from build123d import *

# Parameters (mm, degrees)
F0_W     = 76.2
F0_H     = 50.8
F0_R     = 12.7
F1_DEPTH = 12.7
F2_W     = 6.35
F2_H     = 50.8
F3_DEPTH = 2.54
F5_DEPTH = 58
F6_R     = 3.175
F7_DEPTH = 12.7


# Not quite as in the source:
# - a feature names something its author has since deleted; it is built from what else it names


with BuildPart() as f1:
    # F0 (on Top) → F1 (new body)
    with BuildSketch(Plane.XY):
        with Locations((-0.2381126344, 0.8489250481)):
            Rectangle(F0_W, F0_H)
        Circle(F0_R, mode=Mode.SUBTRACT)
    extrude(amount=F1_DEPTH)

    # F2 (on face) → F3 (cut)
    with BuildSketch(Plane.XY.offset(12.7)):
        with BuildLine():
            Line((6.35, 26.2489250481), (-6.35, 26.2489250481))
            Line((-6.35, 26.2489250481), (-6.35, 10.9985226281))
            ThreePointArc((-6.35, 10.9985226281), (0, 12.7), (6.35, 10.9985226281))
            Line((6.35, 10.9985226281), (6.35, 26.2489250481))
        make_face()
        with BuildLine():
            ThreePointArc((6.35, -10.9985226281), (0, -12.7), (-6.35, -10.9985226281))
            Line((-6.35, -10.9985226281), (-6.35, -24.5510749519))
            Line((-6.35, -24.5510749519), (6.35, -24.5510749519))
            Line((6.35, -24.5510749519), (6.35, -10.9985226281))
        make_face()
        with Locations((-32.6231126344, 0.8489250481)):
            Rectangle(F2_W, F2_H)
    extrude(amount=-F3_DEPTH, mode=Mode.SUBTRACT)

    # F4 (on face) → F5 (cut)
    with BuildSketch(Plane.XZ.offset(24.5510749519)):
        Polygon((32.2451825857, 12.7), (19.5451825857, 12.7), (17.0051825857, 8.3005909488), (34.7851825857, 8.3005909488), align=None)
    extrude(amount=-F5_DEPTH, mode=Mode.SUBTRACT)

    # F6 (on face) → F7 (join)
    with BuildSketch(Plane.YZ.offset(37.8618873656)):
        with Locations((0, 6.35)):
            Circle(F6_R)
    extrude(amount=F7_DEPTH)


solid = f1.part
The listing builds one solid part. Answer for the finished solid, in the listing's coordinates (mm). A direction names the side the tool comes from. Coordinates: 2 decimals unless noted, no trailing zeros. Loops run counter-clockwise (first coordinate to the right, second up) from the corner with the lowest first, then second, coordinate; pieces in that order, holes last.
1) Flat-ended cylindrical pins translate along their axes: pin 1 Ø14 at (x, y) = (2.5, 15) entering from +Z; pin 2 Ø2 at (y, z) = (21.5, 11) entering from +X; pin 3 Ø10 at (x, y) = (-0.5, -19.5) entering from +Z; pin 4 Ø4 at (x, z) = (41, 5.5) entering from +Y (3 decimals). Find the tip coordinate at first contact, or state that the pin passes through.
2) Find section D-D on y = -18. Write down the section's boundary in (x, z).
3) Find section C-C on z = 6.35. Write down the section's boundary in (x, y) (3 decimals).
4) Determine the mould class of faces 1 (the face through (0, 19, 10.16)), 2 (the face through (13, 1, 12.7)), 3 (the face through (50.562, 0, 6)), 4 (the face through (-38.338, 0, 6)) for opening direction X: pulls with the +X half, pulls with the -X half, needs draft (parallel to the pull), parting line crosses it, or undercut.
5) Find the intervals of material crossed by L1, parallel to Y at x = 0, z = 6; L2, parallel to X at y = -21, z = 12; L3, parallel to X at y = 0, z = 4, in increasing order.
6) Find section B-B on y = 0. Write down the section's boundary in (x, z) (3 decimals).
7) Find section A-A on x = 0. Write down the section's boundary in (y, z).
8) A tool of negligible diameter and unlimited length cuts with its end or side. For faces 5 (the face through (18.293, 0.493, 10.531)), 6 (the face through (-1, 26.249, 6)), 7 (the face through (-35.798, 0, 11)), from which of +Z, -Z, +X, -X, +Y, -Y can it reach the whole face along a straight path? Write none if from no direction.
Values:
1. pin 1: stops at z = 12.7
1. pin 2: stops at x = 37.86
1. pin 3: stops at z = 10.16
1. pin 4: stops at y = 3.175
2. outline: (-38.34, 0) - (37.86, 0) - (37.86, 12.7) - (32.25, 12.7) - (34.79, 8.3) - (17.01, 8.3) - (19.55, 12.7) - (6.35, 12.7) - (6.35, 10.16) - (-6.35, 10.16) - (-6.35, 12.7) - (-29.45, 12.7) - (-29.45, 10.16) - (-35.8, 10.16) - (-35.8, 12.7) - (-38.34, 12.7) - close
3. outline: (-38.338, -24.551) - (37.862, -24.551) - (37.862, -3.175) - (50.562, -3.175) - (50.562, 3.175) - (37.862, 3.175) - (37.862, 26.249) - (-38.338, 26.249) - close; hole circle Ø25.4 at (0, 0)
4. face 1: undercut
4. face 2: needs draft
4. face 3: pulls with the +X half
4. face 4: pulls with the -X half
5. L1: y = -24.55 to -12.7, 12.7 to 26.25
5. L2: x = -38.34 to -35.8, -29.45 to -6.35, 6.35 to 19.14, 32.65 to 37.86
5. L3: x = -38.34 to -12.7, 12.7 to 50.56
6. outline: (-38.338, 0) - (-12.7, 0) - (-12.7, 12.7) - (-29.448, 12.7) - (-29.448, 10.16) - (-35.798, 10.16) - (-35.798, 12.7) - (-38.338, 12.7) - close; (12.7, 0) - (37.862, 0) - (37.862, 3.175) - (50.562, 3.175) - (50.562, 9.525) - (37.862, 9.525) - (37.862, 12.7) - (32.245, 12.7) - (34.785, 8.301) - (17.005, 8.301) - (19.545, 12.7) - (12.7, 12.7) - close
7. outline: (-24.55, 0) - (-12.7, 0) - (-12.7, 10.16) - (-24.55, 10.16) - close; (12.7, 0) - (26.25, 0) - (26.25, 10.16) - (12.7, 10.16) - close
8. face 5: +Y, -Y
8. face 6: +Z, -Z, +X, -X, +Y
8. face 7: +Z, +Y, -Y
